Part print with two shaded views. Sizes in mm from the minimum x, y, z corner. A direction names the side the tool comes from. Round coordinates to 2 decimals unless told otherwise and drop trailing zeros. Write each loop counter-clockwise with the first axis right and the second up, starting at its lowest first coordinate (ties: lowest second). Pieces come first, ordered by that corner, then holes. Notation, with made-up numbers: (-32.75, 57) - (17.25, 57) arc R26 cw to (17.25, 81) - close; hole circle Ø11 at (-21, 88). An arc over 180 degrees is marked (long way). Answer as a JSON object with one key per item and string values. Group by question number.
Item 1: Slice it at B-B, the plane y = 60. List the corners of the cut face in (x, z).
Item 2: Slice it at C-C, the plane z = 9. List the corners of the cut face in (x, y).
Item 3: Slice it at D-D, the plane y = 70.5. List the corners of the cut face in (x, z).
Item 4: Which spindle directions (+Z, -Z, +X, -X, +Y, -Y) get a long thin tool onto all of the face, cutting with end or side? Do the marked faces 4, 5 and 6. Say none if no direction does.
Item 5: Flat gauge pins, fed straight in: pin 1 (2.5 mm diameter, centred on x = 37.5, z = 8, fed in from +Y); pin 2 (8 mm diameter, centred on x = 26, y = 36.5, fed in from +Z); pin 3 (1.5 mm diameter, centred on y = 25.5, z = 7, fed in from +X). Where does each tip first touch, or does it go through?
Item 6: Probe line 1 (Y direction, x = 43, z = 0.55); line 2 (Z direction, x = 29.5, y = 67.5); line 3 (Z direction, x = 38.5, y = 28.5). List the from-to ranges inside material, lowest first. Write a range as from..to.
Item 7: Slice it at A-A, the plane x = 43. List the corners of the cut face in (y, z).
Item 8: Two-plate mould, pull along Y, no slides. Class the marked faces 1, 2 and 3: +Y half, -Y half, draft (parallel to the pull), parting line (faces both ways), or undercut.
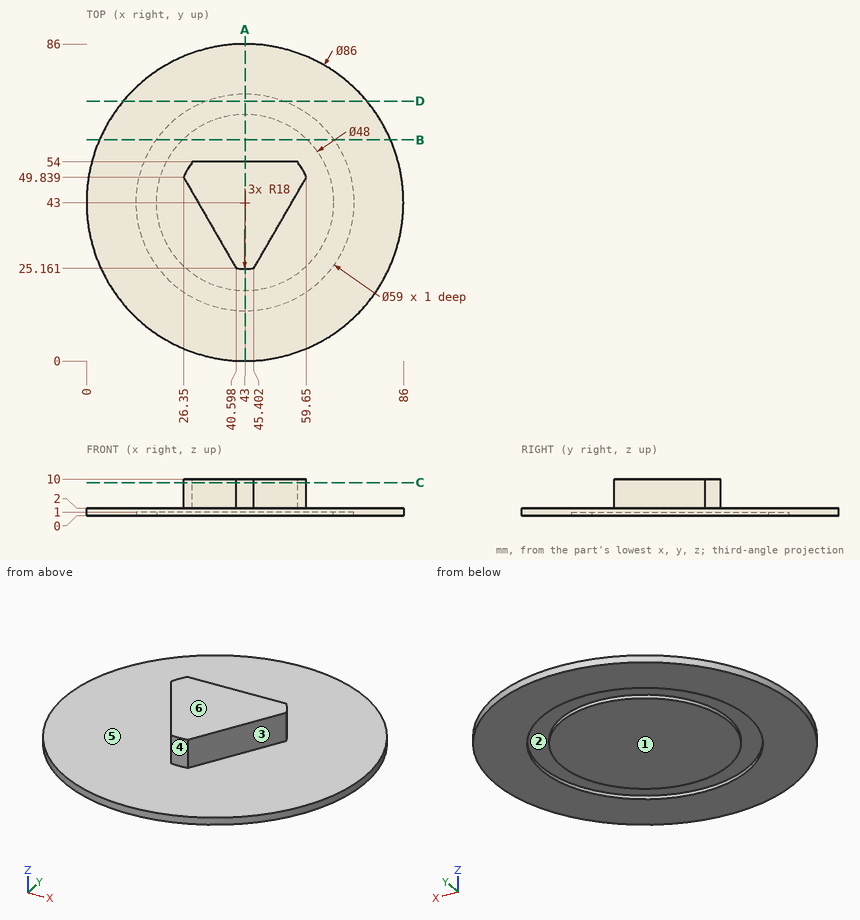
Geometry says:
{
 "1": {"outline": "(3.5, 0) - (18.89, 0) - (18.89, 1) - (26.06, 1) - (26.06, 0) - (59.94, 0) - (59.94, 1) - (67.11, 1) - (67.11, 0) - (82.5, 0) - (82.5, 2) - (3.5, 2) - close"},
 "2": {"outline": "(26.35, 49.84) - (40.6, 25.16) arc R18 ccw to (45.4, 25.16) - (59.65, 49.84) arc R18 ccw to (57.25, 54) - (28.75, 54) arc R18 ccw to start"},
 "3": {"outline": "(9.94, 0) - (32.32, 0) - (32.32, 1) - (53.68, 1) - (53.68, 0) - (76.06, 0) - (76.06, 2) - (9.94, 2) - close"},
 "4": {"face 4": "+Z, -Y", "face 5": "+Z", "face 6": "+Z, +X, -X, +Y, -Y"},
 "5": {"pin 1": "stops at y = 54", "pin 2": "stops at z = 2", "pin 3": "stops at x = 46.03"},
 "6": {"line 1": "y = 0..13.5, 19..67, 72.5..86", "line 2": "z = 1..2", "line 3": "z = 0..2"},
 "7": {"outline": "(0, 0) - (13.5, 0) - (13.5, 1) - (19, 1) - (19, 0) - (67, 0) - (67, 1) - (72.5, 1) - (72.5, 0) - (86, 0) - (86, 2) - (54, 2) - (54, 10) - (25, 10) - (25, 2) - (0, 2) - close"},
 "8": {"face 1": "draft", "face 2": "undercut", "face 3": "-Y half"}
}
